Model file for the job. Use its own axes, mm. A direction names the side the tool comes from. Round coordinates to 2 decimals unless told otherwise and drop trailing zeros. Write each loop counter-clockwise with the first axis right and the second up, starting at its lowest first coordinate (ties: lowest second). Pieces come first, ordered by that corner, then holes. Notation, with made-up numbers: (26, -34.75) - (63, -34.75) arc R32 ccw to (63, -1.75) - close; hole circle Ø9 at (70.25, 4). An arc over 180 degrees is marked (long way). One line per item, written item: value.
Autodesk Inventor part; units mm, degrees
ref_plane "YZ Plane" through (0, 0, 0) normal (1, 0, 0) x (0, 1, 0)
ref_plane "XZ Plane" through (0, 0, 0) normal (0, 1, 0) x (-1, 0, 0)
ref_plane "XY Plane" through (0, 0, 0) normal (0, 0, 1) x (1, 0, 0)
sketch "Sketch1" plane through (0, 0, 0) normal (0, 0, 1) x (1, 0, 0)
  circle A0 centre (0, 0) radius 22.5
  circle A1 centre (-10, 0) radius 1.05
  circle A2 centre (8, 0) radius 0.85
  circle A3 centre (5, -8.6603) radius 1.05
  circle A4 centre (5, 8.6603) radius 1.05
  circle A5 centre (-4, 6.9282) radius 0.85
  circle A6 centre (-4, -6.9282) radius 0.85
  dimension "d0" = 45
  dimension "d1" = 1.7
  dimension "d2" = 2.1
  dimension "d3" = 10
  dimension "d4" = 8
  dimension "d7" = 360
  dimension "d11" = 360
extrude "Extrusion1" add sketch "Sketch1" along normal blind 5
sketch "Sketch2" plane through (0, 0, 5) normal (0, 0, 1) x (1, 0, 0)
  line L0 (-4.1, -4.1) -> (4.1, -4.1)
  line L1 (4.1, -4.1) -> (4.1, 4.1)
  line L2 (4.1, 4.1) -> (-4.1, 4.1)
  line L3 (-4.1, 4.1) -> (-4.1, -4.1)
  line L4 (-4.1, -4.1) -> (4.1, 4.1) construction
  line L5 (4.1, -4.1) -> (-4.1, 4.1) construction
  point P0 (0, 0)
  dimension "d15" = 8.2
  dimension "d16" = 8.2
extrude "Extrusion2" cut sketch "Sketch2" against normal blind 3
sketch "Sketch3" plane through (0, 0, 5) normal (0, 0, 1) x (1, 0, 0)
  line L0 (4.1, 4.1) -> (4.1, -4.1)
  line L1 (-4.1, 4.1) -> (4.1, 4.1)
  line L2 (-4.1, -4.1) -> (-4.1, 4.1)
  line L3 (4.1, -4.1) -> (-4.1, -4.1)
  point P0 (0, 0)
extrude "Extrusion3" add sketch "Sketch3" along normal blind 20 and the other way blind 3
sketch "Sketch4" plane through (0, 0, 25) normal (0, 0, 1) x (1, 0, 0)
  line L0 (-11, 4.1) -> (11, 4.1)
  line L1 (11, 4.1) -> (11, -4.1)
  line L2 (11, -4.1) -> (-11, -4.1)
  line L3 (-11, -4.1) -> (-11, 4.1)
  line L4 (-11, 4.1) -> (11, -4.1) construction
  line L5 (11, 4.1) -> (-11, -4.1) construction
  point P0 (0, 0)
  dimension "d23" = 22
  dimension "d24" = 8.2
extrude "Extrusion4" add sketch "Sketch4" along normal blind 17
sketch "Sketch5" plane through (0, 0, 42) normal (0, 0, 1) x (1, 0, 0)
  line L0 (11, -4.1) -> (11, 4.1)
  line L1 (-11, 1) -> (11, 1)
  line L2 (11, 1) -> (11, -1)
  line L3 (11, -1) -> (-11, -1)
  line L4 (-11, -1) -> (-11, 1)
  line L5 (-11, 1) -> (11, -1) construction
  line L6 (11, 1) -> (-11, -1) construction
  point P0 (0, 0)
  dimension "d27" = 2
extrude "Extrusion5" cut sketch "Sketch5" against normal blind 12
sketch "Sketch6" plane through (-4.1, 4.1, 5) normal (0, 1, 0) x (1, 0, 0)
  circle A0 centre (-0.9, -31) radius 1
  line L0 (-6.9, -20) -> (-6.9, -37)
  line L1 (15.1, -37) -> (-6.9, -37)
  point P0 (4.1, 5)
  dimension "d30" = 6
  dimension "d31" = 6
  dimension "d32" = 2
extrude "Extrusion6" cut sketch "Sketch6" against normal through all
mirror "Mirror1" about plane through (0, 0, 0) normal (1, 0, 0) of "Extrusion6"
fillet "Fillet1" radius 2 8 edges at (11, 2.55, 42) (11, -2.55, 42) (11, 0, 25) (4.1, 0, 25) (-4.1, 0, 25) (-11, 0, 25) (-11, -2.55, 42) (-11, 2.55, 42)
properties part number "WTS_RW_base"
1. Mould opens along X. For faces 1 (the face through (-9, -0.32, 2.46)), 2 (the face through (-10.43, -2.53, 41.4)), 3 (the face through (5, 0, 5)) say: released by +X, released by -X, zero draft, split by the parting line, or undercut.
Report:
face 1: undercut
face 2: released by -X
face 3: zero draft
2. Band-saw the part on D-D on x = -10. Write the cut outline in (y, z).
Report:
outline: (-20.16, 0) - (-1.05, 0) - (-1.05, 5) - (-20.16, 5) - close; (-4.1, 25.27) - (4.1, 25.27) - (4.1, 41.73) - (1, 41.73) - (1, 30) - (-1, 30) - (-1, 41.73) - (-4.1, 41.73) - close; (1.05, 0) - (20.16, 0) - (20.16, 5) - (1.05, 5) - close
3. Band-saw the part on A-A on x = 0. Write the cut outline in (y, z), plus the area to 3 significant figures.
Report:
outline: (-22.5, 0) - (22.5, 0) - (22.5, 5) - (4.1, 5) - (4.1, 42) - (1, 42) - (1, 30) - (-1, 30) - (-1, 42) - (-4.1, 42) - (-4.1, 5) - (-22.5, 5) - close
area: 504 mm²
4. Wall check: probe 1 along X at (y, z) = (3.1, 36); probe 2 along Y at (x, z) = (-5.5, 37.5); probe 3 along Y at (x, z) = (5, 3). Give the ranges that are in metal, low to high. Write a range as [from, to].
Report:
probe 1: [-11, -6], [-4, 4], [6, 11]
probe 2: [-4.1, -1], [1, 4.1]
probe 3: [-21.94, -9.71], [-7.61, 7.61], [9.71, 21.94]
5. Band-saw the part on B-B on x = 5. Write the cut outline in (y, z).
Report:
outline: (-21.94, 0) - (-9.71, 0) - (-9.71, 5) - (-21.94, 5) - close; (-7.61, 0) - (7.61, 0) - (7.61, 5) - (-7.61, 5) - close; (-4.1, 24.67) - (4.1, 24.67) - (4.1, 35) - (1, 35) - (1, 30) - (-1, 30) - (-1, 35) - (-4.1, 35) - close; (-4.1, 37) - (-1, 37) - (-1, 42) - (-4.1, 42) - close; (1, 37) - (4.1, 37) - (4.1, 42) - (1, 42) - close; (9.71, 0) - (21.94, 0) - (21.94, 5) - (9.71, 5) - close
6. Tool access for faces 4 (the face through (0, 1, 36)), 5 (the face through (8, 0, 25)), 6 (the face through (0, 4.1, 27)), 7 (the face through (11, 2, 33)), 8 (the face through (8.785, 0.326, 2.465)): list every direction of +Z, -Z, +X, -X, +Y, -Y with a clear straight run to the whole face (end or side of a thin tool).
Report:
face 4: +Z, +X, -X
face 5: +X, +Y, -Y
face 6: +Z, +X, -X, +Y
face 7: +Z, +X, +Y, -Y
face 8: -Z
7. Band-saw the part on C-C on z = 12. Write the cut outline in (x, y), plus the area to 3 significant figures.
Report:
outline: (-4.1, -4.1) - (4.1, -4.1) - (4.1, 4.1) - (-4.1, 4.1) - close
area: 67.2 mm²
8. Drop flat-ended pins along their axis: pin 1 (11 mm diameter, centred on x = 5.5, z = 18, fed in from -Y); pin 2 (3 mm diameter, centred on x = 8, y = 6, fed in from +Z); pin 3 (6 mm diameter, centred on x = -5.5, z = 38, fed in from +Y). Give the stop position or say it passes through.
Report:
pin 1: y = -4.1
pin 2: z = 5
pin 3: y = 4.1
